Geometry check sheet. Reference: the model listing, model coordinates, mm. A direction names the side the tool comes from. Coordinates: 2 decimals unless noted, no trailing zeros. Loops run counter-clockwise (first coordinate to the right, second up) from the corner with the lowest first, then second, coordinate; pieces in that order, holes last.
from build123d import *

# Parameters (mm, degrees)
OUTBOARD_FOOT_START                 = -6
SKETCH1_W                           = 14
SKETCH1_H                           = 12
SKETCH1_R                           = 1.7
OUTBOARD_FOOT_DEPTH                 = 6
DROP_WEB_START                      = -71
SKETCH2_W                           = 12
SKETCH2_H                           = 12
DROP_WEB_DEPTH                      = 69.5
CROSS_SLOT_BLOCK_START              = -85
SKETCH3_W                           = 40
SKETCH3_H                           = 24
CROSS_SLOT_BLOCK_DEPTH              = 14
X_FLOATING_Y_DRIVEN_SLOT_DEPTH      = 108.763630228
X_FLOATING_Y_DRIVEN_SLOT_DEPTH_BACK = 108.763630228
SKETCH4_W                           = 8
SKETCH4_H                           = 19.02


with BuildPart() as part:
    # Sketch1 → Outboard_Foot (new body)
    with BuildSketch(Plane.XY.offset(OUTBOARD_FOOT_START)):
        with Locations((-37, -20)):
            Rectangle(SKETCH1_W, SKETCH1_H)
        with Locations((-35, -23)):
            Circle(SKETCH1_R, mode=Mode.SUBTRACT)
        with Locations((-35, -17)):
            Circle(SKETCH1_R, mode=Mode.SUBTRACT)
    extrude(amount=OUTBOARD_FOOT_DEPTH)

    # Sketch2 → Drop_Web (add)
    with BuildSketch(Plane.XY.offset(DROP_WEB_START)):
        with Locations((-38, -20)):
            Rectangle(SKETCH2_W, SKETCH2_H)
    extrude(amount=DROP_WEB_DEPTH)

    # Sketch3 → Cross_Slot_Block (add)
    with BuildSketch(Plane.XY.offset(CROSS_SLOT_BLOCK_START)):
        with Locations((-38, -20)):
            Rectangle(SKETCH3_W, SKETCH3_H)
    extrude(amount=CROSS_SLOT_BLOCK_DEPTH)

    # Sketch4 → X_Floating_Y_Driven_Slot (cut, two sides: drawn at the far end of the back side and taken through both)
    with BuildSketch(Plane(origin=(0, 0, 0), x_dir=(0, 0, -1), z_dir=(1, 0, 0)).offset(-X_FLOATING_Y_DRIVEN_SLOT_DEPTH_BACK)):
        with Locations((78, -20)):
            Rectangle(SKETCH4_W, SKETCH4_H)
    extrude(amount=X_FLOATING_Y_DRIVEN_SLOT_DEPTH + X_FLOATING_Y_DRIVEN_SLOT_DEPTH_BACK, mode=Mode.SUBTRACT)


solid = part.part
1) Section check B-B on x = -35. Record the cut outline in (y, z).
Data:
outline: (-32, -85) - (-8, -85) - (-8, -71) - (-14, -71) - (-14, 0) - (-15.3, 0) - (-15.3, -1.5) - (-18.7, -1.5) - (-18.7, 0) - (-21.3, 0) - (-21.3, -1.5) - (-24.7, -1.5) - (-24.7, 0) - (-26, 0) - (-26, -71) - (-32, -71) - close; hole (-29.51, -82) - (-10.49, -82) - (-10.49, -74) - (-29.51, -74) - close
2) Mould release check, pull along X, two halves, no side actions. Record for faces 1 (the flat face through (-38, -32, -78)), 2 (the flat face through (-32, -20, -39)), 3 (the cylindrical face through (-33.38, -16.49, -0.76)), 4 (the cylindrical face through (-36.25, -21.85, -0.76)): +X half, -X half, draft (parallel to the pull), parting line (faces both ways), or undercut.
Data:
face 1: draft
face 2: +X half
face 3: undercut
face 4: undercut
3) Material ranges on probe 1 along X at (y, z) = (-17, -1.1); probe 2 along Z at (x, y) = (-45.5, -16.5); probe 3 along Y at (x, z) = (-35, -0.85), recorded low to high.
Data:
probe 1: x = -44 to -36.7, -33.3 to -30
probe 2: z = -85 to -82, -74 to -71
probe 3: y = -26 to -24.7, -21.3 to -18.7, -15.3 to -14
4) Depth check by flat-ended pin: pin 1 (6 mm diameter, centred on y = -23.5, z = -60.5, fed in from -X); pin 2 (9.5 mm diameter, centred on y = -18.5, z = -34.5, fed in from +X); pin 3 (4 mm diameter, centred on x = -40, z = -41, fed in from +Y). Enter the tip coordinate at first touch or a pass-through.
Data:
pin 1: stops at x = -44
pin 2: stops at x = -32
pin 3: stops at y = -14
5) Section check A-A on y = -11.5. Record the cut outline in (x, z), and give its area (3 significant figures).
Data:
outline: (-58, -85) - (-18, -85) - (-18, -82) - (-58, -82) - close; (-58, -74) - (-18, -74) - (-18, -71) - (-58, -71) - close
area: 240 mm2
6) Section check D-D on z = -53. Record the cut outline in (x, y), and give its area (3 significant figures).
Data:
outline: (-44, -26) - (-32, -26) - (-32, -14) - (-44, -14) - close
area: 144 mm2
7) Section check C-C on y = -17. Record the cut outline in (x, z).
Data:
outline: (-58, -85) - (-18, -85) - (-18, -82) - (-58, -82) - close; (-58, -74) - (-18, -74) - (-18, -71) - (-32, -71) - (-32, -6) - (-30, -6) - (-30, 0) - (-33.3, 0) - (-33.3, -1.5) - (-36.7, -1.5) - (-36.7, 0) - (-44, 0) - (-44, -71) - (-58, -71) - close
8) Access from +Z, -Z, +X, -X, +Y, -Y to the whole of each face (thin tool, end or side, straight path). Record for faces 5 (the flat face through (-30, -20, -3)), 6 (the flat face through (-31, -20, -6)), 7 (the flat face through (-37, -26, -36)), 8 (the flat face through (-35, -17, -1.5)), 9 (the flat face through (-38, -29.51, -78)).
Data:
face 5: +Z, +X, +Y, -Y
face 6: +X, +Y, -Y
face 7: +Z, +X, -X, -Y
face 8: +Z
face 9: +X, -X
